The listing builds one solid part. Answer for the finished solid, in the listing's coordinates (mm). A direction names the side the tool comes from. Round coordinates to 2 decimals unless told otherwise and drop trailing zeros. Write each loop counter-clockwise with the first axis right and the second up, starting at its lowest first coordinate (ties: lowest second). Pieces come first, ordered by that corner, then holes.
Item 1: Find section C-C on x = 15.5. Give the vertices of the cut face in (y, z).
Item 2: Find section D-D on z = 1.5. Give the vertices of the cut face in (x, y), then the cut area to 3 significant figures.
Item 3: Find the intervals of material crossed by probe 1 along X at (y, z) = (1, 0.5); probe 2 along Y at (x, z) = (27, 1); probe 3 along Y at (x, z) = (0.5, 1) (3 decimals), in increasing order.
Item 4: Each of these flat-tipped pins is pushed along its axis until it touches: pin 1 (1.5 mm diameter, centred on y = -4.5, z = 7, fed in from +X); pin 2 (3 mm diameter, centred on y = -10.5, z = 3, fed in from +X); pin 3 (2 mm diameter, centred on x = 22, y = -8.5, fed in from -Z); pin 4 (2 mm diameter, centred on x = 30.5, z = 3, fed in from -Y). Where does it stop, or does it pass through?
Item 5: A tool of negligible diameter and unlimited length cuts with its end or side. For faces 1 (the face through (33, 12, 5)), 2 (the face through (32.5, 0.5, 5.1)), 3 (the face through (1.01, 10.23, 4.93)), 4 (the face through (0, 4.2, 1.6)), from which of +Z, -Z, +X, -X, +Y, -Y can it reach the whole face along a straight path? Write none if from no direction.
Item 6: For a pull along Z with two mould halves and no side action, classify faces 5 (the face through (15.2, -0.4, 0)), 6 (the face through (30.01, 10.27, 4.93)), 7 (the face through (32, 8, 5)) as +Z half, -Z half, draft (parallel to the pull), parting line (faces both ways), or undercut.
Item 7: Find section B-B on y = 7.5. Give the vertices of the cut face in (x, z), then the cut area to 3 significant figures.
Item 8: Find section A-A on z = 5. Give the vertices of the cut face in (x, y), then the cut area to 3 significant figures.
```python
from build123d import *

# Parameters (mm, degrees)
BOSS_EXTRUDE1_DEPTH = 10
CUT_EXTRUDE1_DEPTH  = 41.162171256
SKETCH3_R           = 4
BOSS_EXTRUDE2_DEPTH = 10


with BuildPart() as part:
    # Sketch1 → Boss-Extrude1 (new body)
    with BuildSketch(Plane.XY):
        Polygon((0, 0), (0, 8.5), (2, 8.5), (0, 12), (-3, 12), (-3, -3), (34, -3), (34, 12), (31, 12), (29, 8.5), (31, 8.5), (31, 0), align=None)
    extrude(amount=BOSS_EXTRUDE1_DEPTH)

    # Sketch2 → Cut-Extrude1 (cut, through all)
    with BuildSketch(Plane.ZY.offset(3)):
        with BuildLine():
            Line((8, 5), (8, 3.5))
            ThreePointArc((8, 3.5), (5, 0.5), (2, 3.5))
            Line((2, 3.5), (2, 5))
            ThreePointArc((2, 5), (5, 8), (8, 5))
        make_face()
    extrude(amount=-CUT_EXTRUDE1_DEPTH, mode=Mode.SUBTRACT)

    # Sketch3 → Boss-Extrude2 (add)
    with BuildSketch(Plane.XZ.offset(3)):
        with Locations((15.5, 5)):
            Circle(SKETCH3_R)
    extrude(amount=BOSS_EXTRUDE2_DEPTH)


solid = part.part
```
Check values:
1. outline: (-13, 1) - (-3, 1) - (-3, 0) - (0, 0) - (0, 10) - (-3, 10) - (-3, 9) - (-13, 9) - close
2. outline: (-3, -3) - (13.56, -3) - (13.56, -13) - (17.44, -13) - (17.44, -3) - (34, -3) - (34, 12) - (31, 12) - (29, 8.5) - (31, 8.5) - (31, 0) - (0, 0) - (0, 8.5) - (2, 8.5) - (0, 12) - (-3, 12) - close
2. area: 229 mm2
3. probe 1: x = -3 to 0, 31 to 34
3. probe 2: y = -3 to 0
3. probe 3: y = -3 to 0, 8.5 to 11.125
4. pin 1: stops at x = 19.3
4. pin 2: stops at x = 19.47
4. pin 3: passes through
4. pin 4: stops at y = -3
5. face 1: +Z, -Z, +X, -X, +Y
5. face 2: +X, -X
5. face 3: +Z, -Z, +Y
5. face 4: +Z, -Z
6. face 5: -Z half
6. face 6: draft
6. face 7: undercut
7. outline: (-3, 0) - (0, 0) - (0, 3.34) - (-3, 3.34) - close; (-3, 6.66) - (0, 6.66) - (0, 10) - (-3, 10) - close; (31, 0) - (34, 0) - (34, 3.34) - (31, 3.34) - close; (31, 6.66) - (34, 6.66) - (34, 10) - (31, 10) - close
7. area: 40.1 mm2
8. outline: (-3, -3) - (11.5, -3) - (11.5, -13) - (19.5, -13) - (19.5, -3) - (34, -3) - (34, 0.5) - (31, 0.5) - (31, 0) - (0, 0) - (0, 0.5) - (-3, 0.5) - close; (-3, 8) - (0, 8) - (0, 8.5) - (2, 8.5) - (0, 12) - (-3, 12) - close; (29, 8.5) - (31, 8.5) - (31, 8) - (34, 8) - (34, 12) - (31, 12) - close
8. area: 225 mm2
